```python
from build123d import *

# Parameters (mm, degrees)
F0_W     = 92
F0_H     = 21
F0_W_2   = 86.023346
F0_H_2   = 3
F0_W_3   = 80
F0_W_4   = 86
F0_R     = 1.5
F1_DEPTH = 1


with BuildPart() as f1:
    # F0 (on Front) → F1 (new body)
    with BuildSketch(Plane.XZ):
        Rectangle(F0_W, F0_H)
        with Locations((0, -6)):
            Rectangle(F0_W_2, F0_H_2, mode=Mode.SUBTRACT)
        with Locations((-3, 6)):
            Rectangle(F0_W_3, F0_H_2, mode=Mode.SUBTRACT)
        Rectangle(F0_W_4, F0_H_2, mode=Mode.SUBTRACT)
        with Locations((41.5, 6)):
            Circle(F0_R, mode=Mode.SUBTRACT)
    extrude(amount=F1_DEPTH)


solid = f1.part
```
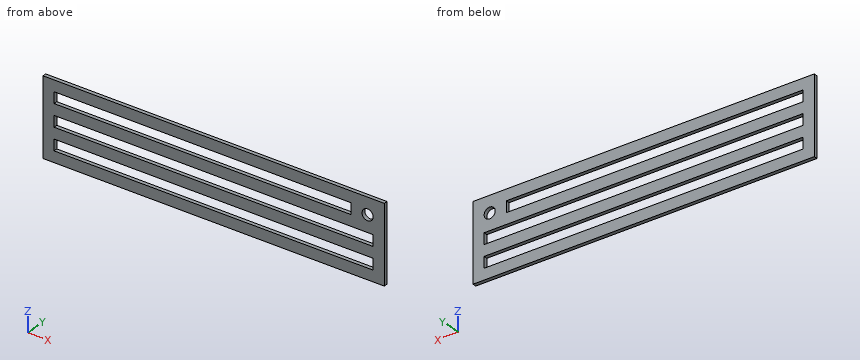
Design review of the part built by this model. Coordinates are the model's own, in mm. Coordinates: 2 decimals unless noted, no trailing zeros. Loops run counter-clockwise (first coordinate to the right, second up) from the corner with the lowest first, then second, coordinate; pieces in that order, holes last. Notation, with made-up numbers: (-39.75, -20) - (-25.75, -20) arc R13 ccw to (-25.75, -8) - close; hole circle Ø11 at (44, 61). An arc over 180 degrees is marked (long way). Use CSV: the item, a comma, the result in double quotes. Start each with the question number.
1) Consider section C-C on y = -0.8. Write out the cut boundary in (x, z).
2) Consider section B-B on x = 35.5. Write out the cut boundary in (y, z), then the cut area to 3 significant figures.
3) Wall thickness on L1, parallel to Z at x = 20.5, y = -0.05; L2, parallel to X at y = -0.15, z = 6.25; L3, parallel to X at y = -0.35, z = 4.75: over which ranges is each line inside the solid? List them lowest first. Write a range as from..to.
4) Consider section A-A on z = 6. Write out the cut boundary in (x, y), then the cut area to 3 significant figures.
Geometry says:
1,outline,"(-46, -10.5) - (46, -10.5) - (46, 10.5) - (-46, 10.5) - close; hole (-43.01, -7.5) - (43.01, -7.5) - (43.01, -4.5) - (-43.01, -4.5) - close; hole (-43, -1.5) - (43, -1.5) - (43, 1.5) - (-43, 1.5) - close; hole (-43, 4.5) - (37, 4.5) - (37, 7.5) - (-43, 7.5) - close; hole circle Ø3 at (41.5, 6)"
2,outline,"(-1, -10.5) - (0, -10.5) - (0, -7.5) - (-1, -7.5) - close; (-1, -4.5) - (0, -4.5) - (0, -1.5) - (-1, -1.5) - close; (-1, 1.5) - (0, 1.5) - (0, 4.5) - (-1, 4.5) - close; (-1, 7.5) - (0, 7.5) - (0, 10.5) - (-1, 10.5) - close"
2,area,"12.0 mm^2"
3,L1,"-10.5..-7.5, -4.5..-1.5, 1.5..4.5, 7.5..10.5"
3,L2,"-46..-43, 37..40.02, 42.98..46"
3,L3,"-46..-43, 37..40.67, 42.33..46"
4,outline,"(-46, -1) - (-43, -1) - (-43, 0) - (-46, 0) - close; (37, -1) - (40, -1) - (40, 0) - (37, 0) - close; (43, -1) - (46, -1) - (46, 0) - (43, 0) - close"
4,area,"9.00 mm^2"
